The listing builds one solid part. Answer for the finished solid, in the listing's coordinates (mm). Coordinates: 2 decimals unless noted, no trailing zeros. Return JSON: item names as keys, results as strings.
```python
from build123d import *

# Parameters (mm, degrees)
CROQUIS1_W                                 = 360
CROQUIS1_H                                 = 35
SALIENTE_EXTRUIR1_DEPTH                    = 4
CROQUIS2_R                                 = 2
CORTAR_EXTRUIR1_DEPTH                      = 5
PERFORADOR_PARA_ROSCAR_PARA_MACHO_DE_ROS_D = 3.3
TALADRO_ROSCADO_M31_D                      = 2.5
CHAFL_N1_SIZE                              = 8
REDONDEO2_R                                = 4


with BuildPart() as part:
    # Croquis1 → Saliente-Extruir1 (new body)
    with BuildSketch(Plane.XY):
        Rectangle(CROQUIS1_W, CROQUIS1_H)
    extrude(amount=SALIENTE_EXTRUIR1_DEPTH)

    # Croquis2 → Cortar-Extruir1 (cut)
    with BuildSketch(Plane.XY.offset(4)):
        with Locations((0, 14)):
            Circle(CROQUIS2_R)
        with Locations((0, -14)):
            Circle(CROQUIS2_R)
        with Locations((161, 14)):
            Circle(CROQUIS2_R)
        with Locations((161, -14)):
            Circle(CROQUIS2_R)
        with Locations((-161, 14)):
            Circle(CROQUIS2_R)
        with Locations((-161, -14)):
            Circle(CROQUIS2_R)
    extrude(amount=-CORTAR_EXTRUIR1_DEPTH, mode=Mode.SUBTRACT)

    # Perforador para roscar para macho de roscar para M41 (through all)
    with Locations(Plane(origin=(-161, 9, 4), x_dir=(1, 0, 0), z_dir=(0, 0, 1))):
        with Locations((0, 0), (0, -18), (161, 0), (161, -18), (322, 0), (322, -18)):
            Hole(PERFORADOR_PARA_ROSCAR_PARA_MACHO_DE_ROS_D / 2)

    # Taladro roscado M31 (through all)
    with Locations(Plane.XY.offset(4)):
        with Locations((-170, 0), (-110, 0), (-50, 0), (50, 0), (110, 0), (170, 0)):
            Hole(TALADRO_ROSCADO_M31_D / 2)

    # Chaflán1
    chafl_n1_edges = [part.edges().sort_by_distance(p)[0] for p in [
        (180, -17.5, 2),
        (-180, -17.5, 2),
        (-180, 17.5, 2),
        (180, 17.5, 2),
    ]]
    chamfer(chafl_n1_edges, length=CHAFL_N1_SIZE)

    # Redondeo2
    redondeo2_edges = [part.edges().sort_by_distance(p)[0] for p in [
        (180, 9.5, 2),
        (180, -9.5, 2),
        (-172, -17.5, 2),
        (172, -17.5, 2),
        (-172, 17.5, 2),
        (172, 17.5, 2),
        (-180, 9.5, 2),
        (-180, -9.5, 2),
    ]]
    fillet(redondeo2_edges, radius=REDONDEO2_R)


solid = part.part
```
Item 1: The part is cut by section A-A on z = 0.8. Count the separate pieces of the cut face and the enclosed holes in it, plus the area to 3 significant figures.
Answer list:
{"separate pieces": "1", "enclosed holes": "18", "area": "12,300 mm2"}
Item 2: A flat-ended cylindrical pin translates along its axis: pin 1 (1.5 mm diameter, centred on x = 170, y = 0, fed in from +Z). Find the tip coordinate at first contact, or state that the pin passes through.
Answer list:
{"pin 1": "through"}
Item 3: Find the intervals of material crossed by probe 1 along Y at (x, z) = (0, 2.7); probe 2 along Y at (x, z) = (-50, 1.55); probe 3 along X at (y, z) = (8.5, 3), in increasing order.
Answer list:
{"probe 1": "-17.5 to -16, -12 to -10.65, -7.35 to 7.35, 10.65 to 12, 16 to 17.5", "probe 2": "-17.5 to -1.25, 1.25 to 17.5", "probe 3": "-179.95 to -162.57, -159.43 to -1.57, 1.57 to 159.43, 162.57 to 179.95"}
